Autodesk Inventor part; units mm, degrees
ref_plane "Конечная плоскость" through (0, 0, 1010) normal (0, 0, 1) x (1, 0, 0)
ref_plane "YZ Plane" through (0, 0, 0) normal (1, 0, 0) x (0, 1, 0)
ref_plane "XZ Plane" through (0, 0, 0) normal (0, 1, 0) x (-1, 0, 0)
sketch "Поручень" plane through (0, 0, 0) normal (0, 0, 1) x (1, 0, 0)
  line L0 (20.3655, -7.6059) -> (20.3655, -0.2092)
  line L1 (20.3655, -0.2092) -> (-19.6345, -0.2092)
  line L2 (-19.6345, -0.2092) -> (-19.6345, -7.6059)
  line L3 (-19.6345, -7.6059) -> (-30.865, -7.6059)
  line L4 (-30.865, -7.6059) -> (-30.865, -5.9622)
  line L5 (-30.865, -5.9622) -> (-32.5087, -5.9622)
  line L6 (-32.5087, -5.9622) -> (-32.5087, 0.6126)
  arc A0 (-30.367, 4.2203) -> (-32.5087, 0.6126) centre (-28.3995, 0.6126) ccw
  arc A1 (-30.367, 4.2203) -> (-30.2973, 18.6123) centre (-34.302, 11.4355) ccw
  arc A2 (-24.2902, 41.7054) -> (-30.2973, 18.6123) centre (-24.2902, 29.3776) ccw
  line L7 (-24.2902, 41.7054) -> (-24.2902, 42.9382)
  arc A3 (25.0211, 42.9382) -> (-24.2902, 42.9382) centre (0.3655, 2.9211) ccw
  line L8 (25.0211, 42.9382) -> (25.0211, 41.7054)
  arc A4 (31.0282, 18.6123) -> (25.0211, 41.7054) centre (25.0211, 29.3776) ccw
  arc A5 (31.0282, 18.6123) -> (31.0979, 4.2203) centre (35.033, 11.4355) ccw
  arc A6 (33.2397, 0.6126) -> (31.0979, 4.2203) centre (29.1304, 0.6126) ccw
  line L9 (33.2397, 0.6126) -> (33.2397, -5.9622)
  line L10 (33.2397, -5.9622) -> (31.596, -5.9622)
  line L11 (31.596, -5.9622) -> (31.596, -7.6059)
  line L12 (31.596, -7.6059) -> (20.3655, -7.6059)
  point P0 (0.3655, -0.2092)
  point P1 (0.3655, -7.6059)
sketch "Эскиз" plane through (0, 0, 0) normal (0, 0, 1) x (1, 0, 0)
  line L0 (20, 0) -> (20, 7.3967)
  line L1 (20, 7.3967) -> (-20, 7.3967)
  line L2 (-20, 7.3967) -> (-20, 0)
  line L3 (-20, 0) -> (-31.2305, 0)
  line L4 (-31.2305, 0) -> (-31.2305, 1.6437)
  line L5 (-31.2305, 1.6437) -> (-32.8742, 1.6437)
  line L6 (-32.8742, 1.6437) -> (-32.8742, 8.2186)
  arc A0 (-30.7325, 11.8262) -> (-32.8742, 8.2186) centre (-28.7649, 8.2186) ccw
  arc A1 (-30.7325, 11.8262) -> (-30.6628, 26.2183) centre (-34.6675, 19.0415) ccw
  arc A2 (-24.6557, 49.3113) -> (-30.6628, 26.2183) centre (-24.6557, 36.9835) ccw
  line L7 (-24.6557, 49.3113) -> (-24.6557, 50.5441)
  arc A3 (24.6557, 50.5441) -> (-24.6557, 50.5441) centre (0, 10.527) ccw
  line L8 (24.6557, 50.5441) -> (24.6557, 49.3113)
  arc A4 (30.6628, 26.2183) -> (24.6557, 49.3113) centre (24.6557, 36.9835) ccw
  arc A5 (30.6628, 26.2183) -> (30.7325, 11.8262) centre (34.6675, 19.0415) ccw
  arc A6 (32.8742, 8.2186) -> (30.7325, 11.8262) centre (28.7649, 8.2186) ccw
  line L9 (32.8742, 8.2186) -> (32.8742, 1.6437)
  line L10 (32.8742, 1.6437) -> (31.2305, 1.6437)
  line L11 (31.2305, 1.6437) -> (31.2305, 0)
  line L12 (31.2305, 0) -> (20, 0)
  point P0 (0, 0)
ref_plane "Начальная плоскость" through (0, 0, 0) normal (0, 0, 1) x (1, 0, 0)
ref_plane "РабПлоскость2" through (0, 0, 1010) normal (0, 0, 1) x (1, 0, 0)
extrude "Тело" add sketch "Эскиз" along normal up to surface (1010 mm away) from surface at 0
ref_plane "Конечная плоскость" through (0, 0, 1010) normal (0, 0, 1) x (1, 0, 0)
equation "\"ШИРИНА\" = 75"
equation "\"ТОЛЩВЫС\" = 58"
equation "\"СЕЧЕНИЕ_СМЕЩ\" = 0"
equation "\"G_OFFSET_END\" = 0"
equation "\"G_OFFSET_START\" = 0"
properties part number "Поручень" material "Древесина (дуб)"
The listing builds one solid part. Answer for the finished solid, in the listing's coordinates (mm). A direction names the side the tool comes from. Coordinates: 2 decimals unless noted, no trailing zeros. Write each loop counter-clockwise with the first axis right and the second up, starting at its lowest first coordinate (ties: lowest second). Pieces come first, ordered by that corner, then holes. Notation, with made-up numbers: M 76.25,3 L 117.25,3 A31 ccw 117.25,36 Z; hole C 10,77 d11. An arc over 180 degrees is marked long. Put each result on its own line as item: value. Start each with the question number.
1. A cutting plane is placed at B-B on x = 11.5. Write down the section's boundary in (y, z), then the cut area to 3 significant figures.
2. A cutting plane is placed at A-A on z = 371.5. Write down the section's boundary in (x, y).
3. Which of the six approach directions +Z, -Z, +X, -X, +Y, -Y give full straight-line access (tool end or side, diameter ignored) to faces 1 (the flat face through (0, 7.397, 498)), 2 (the flat face through (-1, 29, 0))?
4. Consider line 1 (Y direction, x = -2.5, z = 714); line 2 (X direction, y = 9, z = 526.5); line 3 (X direction, y = 5.5, z = 936.5). Determine where each line is inside the solid, lowest interval first. Write a range as from..to.
5. Flat-ended cylindrical pins translate along their axes: P1, Ø6, axis at y = 41.5, z = 110.5, coming from the -X side; P2, Ø2, axis at y = 2.5, z = 750.5, coming from the -X side; P3, Ø1.8, axis at y = 0.5, z = 294.5, coming from the +X side; P4, Ø2, axis at x = -6.5, y = 39, coming from the -Z side. Find the tip coordinate at first contact, or state that the pin passes through.
Resolved:
1. outline: M 7.4,0 L 56.1,0 L 56.1,1010 L 7.4,1010 Z
1. area: 49,200 mm2
2. outline: M -32.87,1.64 L -31.23,1.64 L -31.23,0 L -20,0 L -20,7.4 L 20,7.4 L 20,0 L 31.23,0 L 31.23,1.64 L 32.87,1.64 L 32.87,8.22 A4.11 ccw 30.73,11.83 A8.22 cw 30.66,26.22 A12.33 ccw 24.66,49.31 L 24.66,50.54 A47 ccw -24.66,50.54 L -24.66,49.31 A12.33 ccw -30.66,26.22 A8.22 cw -30.73,11.83 A4.11 ccw -32.87,8.22 Z
3. face 1: +Z, -Z, -Y
3. face 2: -Z, +X, -X, +Y, -Y
4. line 1: y = 7.4..57.46
4. line 2: x = -32.8..32.8
4. line 3: x = -32.87..-20, 20..32.87
5. P1: stops at x = -36.89
5. P2: stops at x = -32.87
5. P3: stops at x = 31.23
5. P4: stops at z = 0
